Verification items for this drawing (mm, ordinates from the low corner). Give positions to 0.01 mm unless a question says otherwise; leave off trailing zeros. Loops run counter-clockwise (first coordinate to the right, second up) from the corner with the lowest first, then second, coordinate; pieces in that order, holes last. Notation, with made-up numbers: (49, 31.5) -> (69, 31.5) arc R23 ccw to (69, 54.5) -> close; hole circle Ø6 at (1.5, 43.5). An arc over 180 degrees is marked (long way). Answer as a JSON object with one key per item and string values.
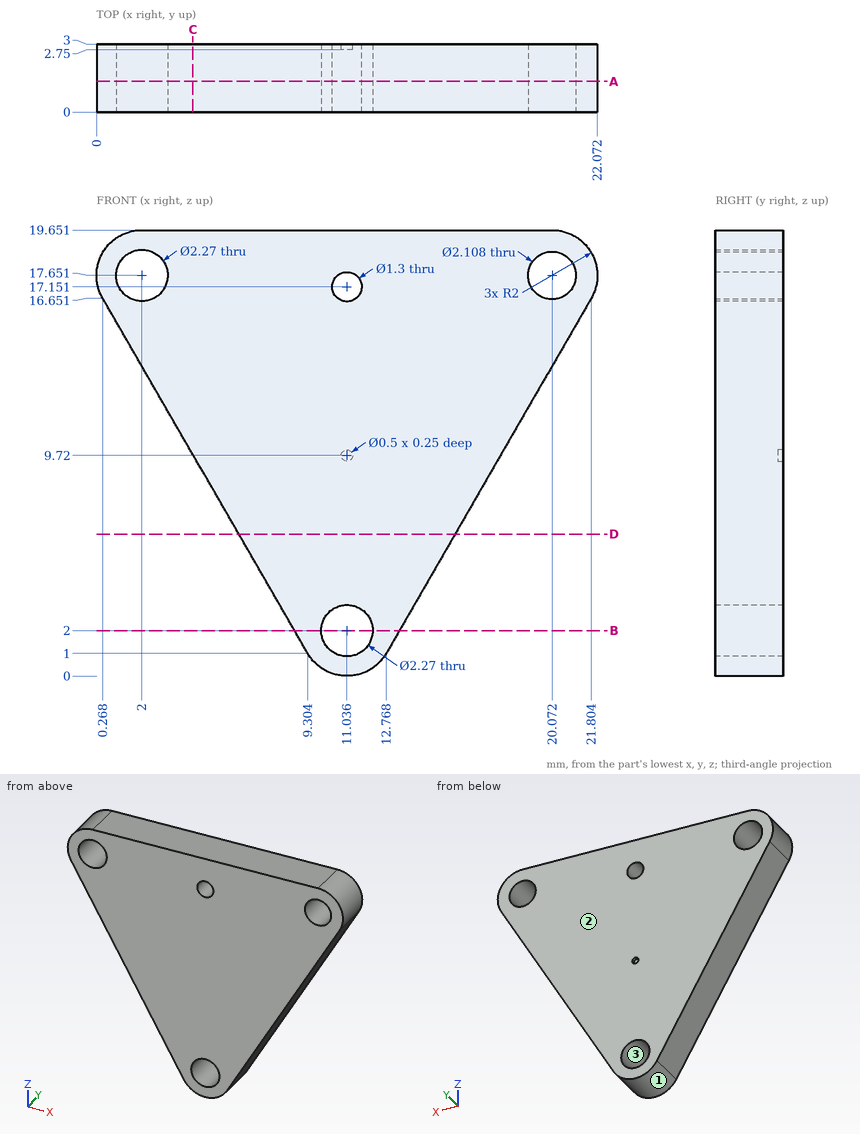
1) Section check D-D on z = 6.25. Record the cut outline in (x, y).
Geometry check:
{"outline": "(6.27, 0) -> (15.8, 0) -> (15.8, 3) -> (6.27, 3) -> close"}
2) Draft check along X on the marked faces 1, 2 and 3. Enter one of: pulls with the +X half, pulls with the -X half, needs draft (parallel to the pull), parting line crosses it, or undercut.
Geometry check:
{"face 1": "parting line crosses it", "face 2": "needs draft", "face 3": "undercut"}
3) Material ranges on line 1 along X through (y, z) = (1.6, 17) (1 decimal); line 2 along X through (y, z) = (1.15, 2.25); line 3 along Z through (x, y) = (11.75, 0.65), recorded low to high. Write a range as from..to.
Geometry check:
{"line 1": "x = 0.1..1.1, 2.9..10.4, 11.7..19.2, 20.9..22", "line 2": "x = 8.58..9.93, 12.14..13.49", "line 3": "z = 0.13..1.12, 2.88..19.65"}
4) Section check A-A on y = 1.35. Count the separate pieces of the cut face and the enclosed holes in it.
Geometry check:
{"separate pieces": "1", "enclosed holes": "4"}
5) Section check B-B on z = 2. Record the cut outline in (x, y) (1 decimal).
Geometry check:
{"outline": "(8.7, 0) -> (9.9, 0) -> (9.9, 3) -> (8.7, 3) -> close; (12.2, 0) -> (13.3, 0) -> (13.3, 3) -> (12.2, 3) -> close"}
6) Section check C-C on x = 4.25. Record the cut outline in (y, z), plus the area to 3 significant figures.
Geometry check:
{"outline": "(0, 9.75) -> (3, 9.75) -> (3, 19.65) -> (0, 19.65) -> close", "area": "29.7 mm2"}
7) Depth check by flat-ended pin: P1, Ø2, axis at x = 11.04, z = 2, coming from the -Y side; P2, Ø1, axis at x = 12.5, y = 2.5, coming from the -Z side. Enter the tip coordinate at first touch or a pass-through.
Geometry check:
{"P1": "passes through", "P2": "stops at z = 0.25"}
